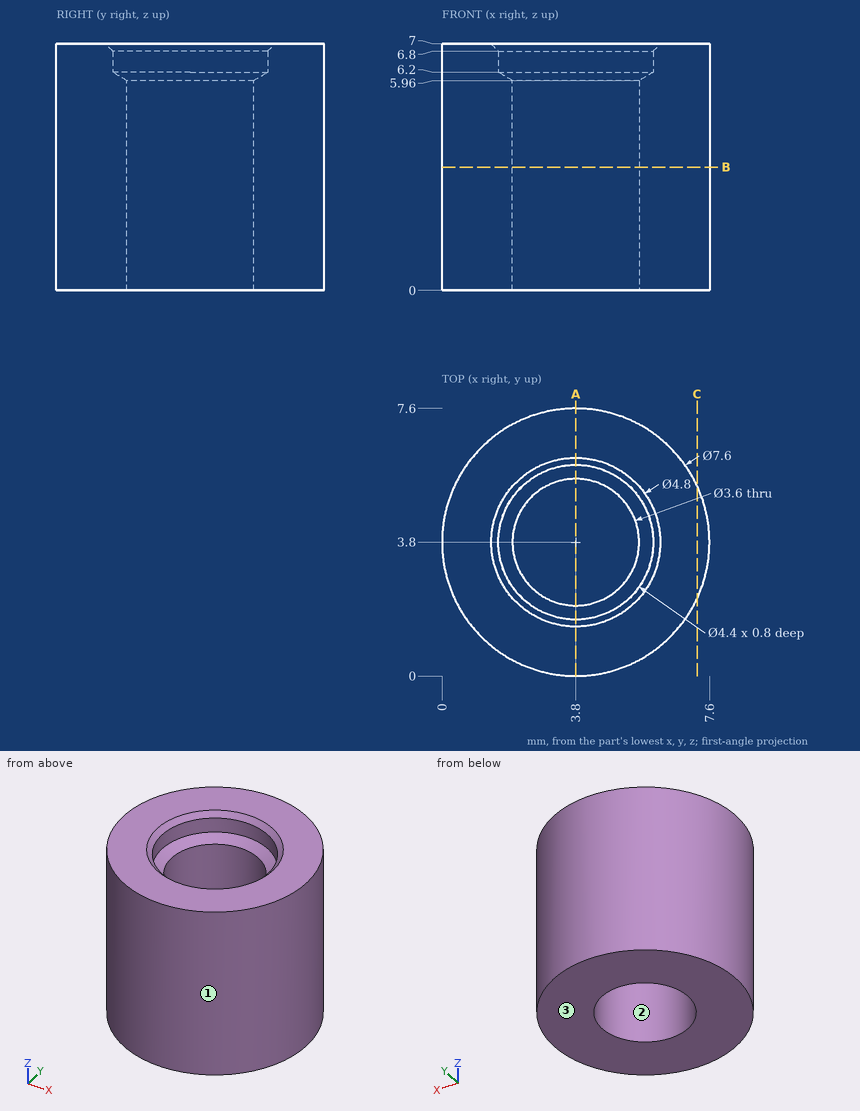
For this review, use the dimensioned drawing (mm, ordinates from the lowest corner) and the shaded views. Round coordinates to 2 decimals unless told otherwise and drop trailing zeros. Write each loop counter-clockwise with the first axis right and the second up, starting at its lowest first coordinate (ties: lowest second). Pieces come first, ordered by that corner, then holes. Notation, with made-up numbers: (-13.5, 87.5) - (25.5, 87.5) arc R17 ccw to (25.5, 94.5) - close; hole circle Ø6 at (30.5, 33.5). An arc over 180 degrees is marked (long way). One line per item, written item: value. Start each with the question number.
1. Consider section C-C on x = 7.25. Write out the cut boundary in (y, z).
2. Clearance check with a flat-ended pin moving along its axis: P1, Ø1.5, axis at x = 6, z = 4.5, coming from the -Y side. State where the tip first meets the part, or that it passes through.
3. Consider section A-A on x = 3.8. Write out the cut boundary in (y, z), and give its area (3 significant figures).
4. Consider section B-B on z = 3.5. Write out the cut boundary in (x, y), and give its area (3 significant figures).
5. To check wall thickness, follow L1, parallel to Y at x = 3.8, z = 6.5; L2, parallel to Y at x = 3.8, z = 3. State the ranges of each line that lie inside material, in increasing order. Write a range as from..to.
6. The part is to be moulded in two halves that separate along Y. For the marked faces 1, 2 and 3, say which applies: released by +Y, released by -Y, zero draft, split by the parting line, or undercut.
Checks:
1. outline: (2.21, 0) - (5.39, 0) - (5.39, 7) - (2.21, 7) - close
2. P1: stops at y = 0.29
3. outline: (0, 0) - (2, 0) - (2, 5.96) - (1.6, 6.2) - (1.6, 6.8) - (1.4, 7) - (0, 7) - close; (5.6, 0) - (7.6, 0) - (7.6, 7) - (6.2, 7) - (6, 6.8) - (6, 6.2) - (5.6, 5.96) - close
3. area: 27.2 mm^2
4. outline: circle Ø7.6 at (3.8, 3.8); hole circle Ø3.6 at (3.8, 3.8)
4. area: 35.2 mm^2
5. L1: y = 0..1.6, 6..7.6
5. L2: y = 0..2, 5.6..7.6
6. face 1: split by the parting line
6. face 2: undercut
6. face 3: zero draft
